```python
from build123d import *

# Parameters (mm, degrees)
BOSS_EXTRUDE1_DEPTH = 3


with BuildPart() as part:
    # Sketch1 → Boss-Extrude1 (new body)
    with BuildSketch(Plane(origin=(0, 0, 0), x_dir=(1, 0, 0), z_dir=(0, 1, 0))):
        Polygon((-66.5, 46), (-66.5, 31), (-62.5, 31), (-62.5, 21), (-66.5, 21), (-66.5, 6), (-62.5, 6), (-62.5, -9), (-66.5, -9), (-66.5, -24), (-62.5, -24), (-62.5, -34), (-66.5, -34), (-66.5, -49), (-62.5, -49), (-62.5, -59), (-62.5, -64), (-57.5, -64), (-47.5, -64), (-47.5, -68), (-32.5, -68), (-32.5, -64), (-22.5, -64), (-22.5, -68), (-7.5, -68), (-7.5, -64), (7.5, -64), (7.5, -68), (22.5, -68), (22.5, -64), (32.5, -64), (32.5, -68), (47.5, -68), (47.5, -64), (57.5, -64), (62.5, -64), (62.5, -59), (62.5, -49), (66.5, -49), (66.5, -34), (62.5, -34), (62.5, -24), (66.5, -24), (66.5, -9), (62.5, -9), (62.5, 6), (66.5, 6), (66.5, 21), (62.5, 21), (62.5, 31), (66.5, 31), (66.5, 46), (62.5, 46), (62.5, 56), (62.5, 61), (57.5, 61), (47.5, 61), (47.5, 65), (32.5, 65), (32.5, 61), (22.5, 61), (22.5, 65), (7.5, 65), (7.5, 61), (-7.5, 61), (-7.5, 65), (-22.5, 65), (-22.5, 61), (-32.5, 61), (-32.5, 65), (-47.5, 65), (-47.5, 61), (-57.5, 61), (-62.5, 61), (-62.5, 56), (-62.5, 46), align=None)
        with BuildLine():
            Line((-35, 50), (-35, -50))
            ThreePointArc((-35, -50), (-40, -55), (-45, -50))
            Line((-45, -50), (-45, 50))
            ThreePointArc((-45, 50), (-40, 55), (-35, 50))
        make_face(mode=Mode.SUBTRACT)
        with BuildLine():
            Line((-10, 50), (-10, -50))
            ThreePointArc((-10, -50), (-15, -55), (-20, -50))
            Line((-20, -50), (-20, 50))
            ThreePointArc((-20, 50), (-15, 55), (-10, 50))
        make_face(mode=Mode.SUBTRACT)
        with BuildLine():
            Line((10, 50), (10, -50))
            ThreePointArc((10, -50), (15, -55), (20, -50))
            Line((20, -50), (20, 50))
            ThreePointArc((20, 50), (15, 55), (10, 50))
        make_face(mode=Mode.SUBTRACT)
        with BuildLine():
            Line((35, 50), (35, -50))
            ThreePointArc((35, -50), (40, -55), (45, -50))
            Line((45, -50), (45, 50))
            ThreePointArc((45, 50), (40, 55), (35, 50))
        make_face(mode=Mode.SUBTRACT)
    extrude(amount=BOSS_EXTRUDE1_DEPTH)


solid = part.part
```
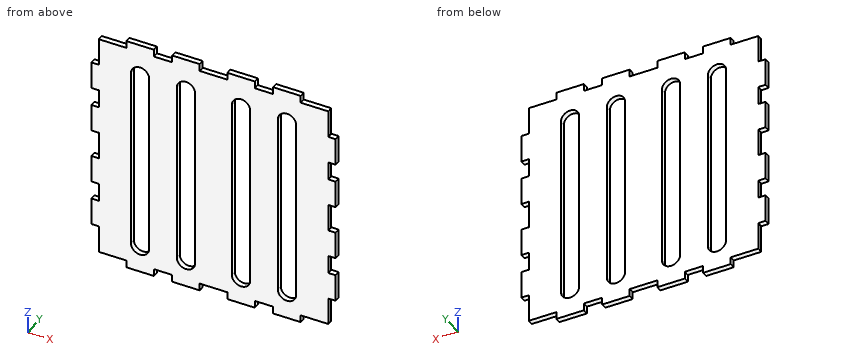
Design review of the part built by this model. Coordinates are the model's own, in mm. Coordinates: 2 decimals unless noted, no trailing zeros. Write each loop counter-clockwise with the first axis right and the second up, starting at its lowest first coordinate (ties: lowest second). Pieces come first, ordered by that corner, then holes. Notation, with made-up numbers: M 40,5.25 L 71,5.25 A22 ccw 71,24.25 Z; hole C 80.25,-35.5 d2. An arc over 180 degrees is marked long. Answer as a JSON object with one key per item and string values.
Item 1: Insertion check: pin 1 Ø0.9 at (y, z) = (1, 55) entering from -X; pin 2 Ø1.5 at (x, y) = (29, 2) entering from -Z; pin 3 Ø1.5 at (x, y) = (-64, 1.5) entering from +Z. Each pin has a flat end and moves straight along its axis. Give the tip position at first contact, or say it passes through.
Outcome:
{"pin 1": "x = -62.5", "pin 2": "z = -61", "pin 3": "z = 49"}
Item 2: Add section C-C, the plane y = 1.1. State how many separate pieces and enclosed holes the cut face has, and give its area (3 significant figures).
Outcome:
{"separate pieces": "1", "enclosed holes": "4", "area": "12,300 mm²"}
Item 3: Wall thickness on probe 1 along X at (y, z) = (1.3, 44); probe 2 along X at (y, z) = (0.9, 1.5); probe 3 along Z at (x, y) = (58, 1.5): over which ranges is each line inside the solid? List them lowest first.
Outcome:
{"probe 1": "-66.5 to -45, -35 to -20, -10 to 10, 20 to 35, 45 to 66.5", "probe 2": "-62.5 to -45, -35 to -20, -10 to 10, 20 to 35, 45 to 62.5", "probe 3": "-61 to 64"}
Item 4: Add section D-D, the plane x = 39. Give the boundary of the cut face in (y, z), and give its area (3 significant figures).
Outcome:
{"outline": "M 0,-65 L 3,-65 L 3,-54.9 L 0,-54.9 Z; M 0,54.9 L 3,54.9 L 3,68 L 0,68 Z", "area": "69.6 mm²"}
Item 5: Add section B-B, the plane z = 15.5. Give the boundary of the cut face in (x, y), and give its area (3 significant figures).
Outcome:
{"outline": "M -66.5,0 L -45,0 L -45,3 L -66.5,3 Z; M -35,0 L -20,0 L -20,3 L -35,3 Z; M -10,0 L 10,0 L 10,3 L -10,3 Z; M 20,0 L 35,0 L 35,3 L 20,3 Z; M 45,0 L 66.5,0 L 66.5,3 L 45,3 Z", "area": "279 mm²"}
Item 6: Add section A-A, the plane x = 15. Give the boundary of the cut face in (y, z).
Outcome:
{"outline": "M 0,-65 L 3,-65 L 3,-55 L 0,-55 Z; M 0,55 L 3,55 L 3,68 L 0,68 Z"}
